from build123d import *

# Parameters (mm, degrees)
SKETCH_1_R          = 10.5
EXTRUDE_1_DEPTH     = 80
SKETCH_2_R          = 2.649752209
EXTRUDE_2_DEPTH     = 100
SKETCH_3_R          = 10.5
SKETCH_3_R_2        = 8
CUT_EXTRUDE_1_DEPTH = 181.61146143


with BuildPart() as part:
    # 草图1 → 凸台-拉伸1 (new body)
    with BuildSketch(Plane(origin=(0, 0, 0), x_dir=(1, 0, 0), z_dir=(0, 1, 0))):
        with Locations(Location((0, 0, 0), (0, 0, 270))):
            Circle(SKETCH_1_R)
    extrude(amount=EXTRUDE_1_DEPTH)

    # 草图2 → 凸台-拉伸2 (add)
    with BuildSketch(Plane(origin=(0, 80, 0), x_dir=(1, 0, 0), z_dir=(0, 1, 0))):
        with Locations(Location((-3.354877279, -0.090103274, 0), (0, 0, 90))):
            Circle(SKETCH_2_R)
        with Locations(Location((3.354877279, -0.090103274, 0), (0, 0, 90))):
            Circle(SKETCH_2_R)
    extrude(amount=EXTRUDE_2_DEPTH)

    # 草图3 → 切除-拉伸1 (cut, through all)
    with BuildSketch(Plane.XZ):
        Circle(SKETCH_3_R)
        with Locations(Location((0, 0, 0), (0, 0, 270))):
            Circle(SKETCH_3_R_2, mode=Mode.SUBTRACT)
    extrude(amount=-CUT_EXTRUDE_1_DEPTH, mode=Mode.SUBTRACT)


solid = part.part
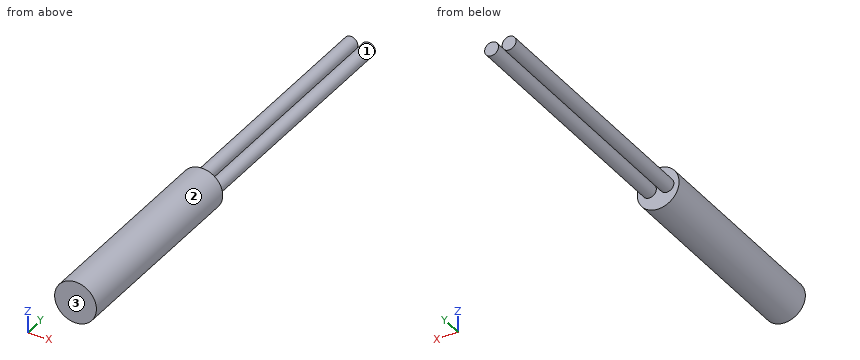
Here's how the part is built. I have some questions about the finished solid (model axes, mm). Face numbers are marked on the shaded views. Give positions to 0.01 mm unless a question says otherwise; leave off trailing zeros. Loops run counter-clockwise (first coordinate to the right, second up) from the corner with the lowest first, then second, coordinate; pieces in that order, holes last. Notation, with made-up numbers: (-36, -20) -> (-6, -20) arc R33 ccw to (-6, 15) -> close; hole circle Ø9 at (57, 87.5). An arc over 180 degrees is marked (long way). Answer as a JSON object with one key per item and string values. Group by question number.
Item 1: Imagine slicing it at B-B on y = 165. Write out the boundary of the cut face in (x, z), then the cut area to 3 significant figures.
Item 2: I need wall thicknesses on L1, parallel to X at y = 166.5, z = 0.5; L2, parallel to Y at x = -4.5, z = 5.75; L3, parallel to X at y = 137, z = -1.5. Which ranges of each line are inside material? Lowest first, please.
Item 3: Imagine slicing it at A-A on z = -0.5. Write out the boundary of the cut face in (x, y), then the cut area to 3 significant figures.
Item 4: Will these pins go through, and if not, where does the flat tip stop? pin 1 (6 mm diameter, centred on y = 104, z = 4.5, fed in from +X); pin 2 (1.5 mm diameter, centred on x = -5, y = 160.5, fed in from -Z); pin 3 (4 mm diameter, centred on x = -3, z = -5, fed in from +Y).
Item 5: Imagine slicing it at C-C on y = 38.5. Write out the boundary of the cut face in (x, z), then the cut area to 3 significant figures.
Item 6: Thinking about a two-plate mould opening in X: for the marked faces 1, 2 and 3, which applies, pulls with the +X half, pulls with the -X half, needs draft (parallel to the pull), parting line crosses it, or undercut?
Answer list:
{
 "1": {"outline": "circle Ø5.3 at (-3.35, 0.09); circle Ø5.3 at (3.35, 0.09)", "area": "44.1 mm2"},
 "2": {"L1": "x = -5.97 to -0.74, 0.74 to 5.97", "L2": "y = 0 to 80", "L3": "x = -5.47 to -1.24, 1.24 to 5.47"},
 "3": {"outline": "(-7.98, 0) -> (7.98, 0) -> (7.98, 80) -> (5.94, 80) -> (5.94, 180) -> (0.77, 180) -> (0.77, 80) -> (-0.77, 80) -> (-0.77, 180) -> (-5.94, 180) -> (-5.94, 80) -> (-7.98, 80) -> close", "area": "2,310 mm2"},
 "4": {"pin 1": "stops at x = 5.6", "pin 2": "stops at z = -2.4", "pin 3": "stops at y = 80"},
 "5": {"outline": "circle Ø16 at (0, 0)", "area": "201 mm2"},
 "6": {"face 1": "undercut", "face 2": "parting line crosses it", "face 3": "needs draft"}
}
